Can you work these out from the model? Positions are in its coordinate system, mm. A direction names the side the tool comes from. Round coordinates to 2 decimals unless told otherwise and drop trailing zeros. Loops run counter-clockwise (first coordinate to the right, second up) from the corner with the lowest first, then second, coordinate; pieces in that order, holes last. Notation, with made-up numbers: (-13.5, 20.25) -> (-7.5, 20.25) arc R20 ccw to (-7.5, 57.25) -> close; hole circle Ø2 at (41, 10.5). An arc over 180 degrees is marked (long way). Use a Markdown table: item, result.
from build123d import *

# Parameters (mm, degrees)
SALIENTE_EXTRUIR1_DEPTH      = 6
SALIENTE_EXTRUIR1_DEPTH_BACK = 6
CROQUIS3_R                   = 2.5
SALIENTE_EXTRUIR2_DEPTH      = 4.5
CROQUIS4_R                   = 2.4
SALIENTE_EXTRUIR5_DEPTH      = 7.5
CORTAR_EXTRUIR1_DEPTH        = 3.5


with BuildPart() as part:
    # Croquis1 → Saliente-Extruir1 (new, two sides: drawn at the far end of the back side and taken through both)
    with BuildSketch(Plane.XY.offset(-SALIENTE_EXTRUIR1_DEPTH_BACK)):
        Polygon((-11.5, 7), (-16.5, 7), (-16.5, 4.5), (-11.5, 4.5), (-11.5, -11.5), (11.5, -11.5), (11.5, 4.5), (16.5, 4.5), (16.5, 7), (11.5, 7), (11.5, 11.5), (-11.5, 11.5), align=None)
    extrude(amount=SALIENTE_EXTRUIR1_DEPTH + SALIENTE_EXTRUIR1_DEPTH_BACK)

    # Croquis3 → Saliente-Extruir2 (add)
    with BuildSketch(Plane(origin=(0, 11.5, 0), x_dir=(1, 0, 0), z_dir=(0, 1, 0))):
        with BuildLine():
            Line((0.5, 2.5), (-0.045643943, 2.5))
            ThreePointArc((-0.045643943, 2.5), (-11.5, 0), (-0.045643943, -2.5))
            Line((-0.045643943, -2.5), (0.5, -2.5))
            ThreePointArc((0.5, -2.5), (3, 0), (0.5, 2.5))
        make_face()
        with Locations(Location((-5.5, 0, 0), (0, 0, 270))):
            Circle(CROQUIS3_R, mode=Mode.SUBTRACT)
    extrude(amount=SALIENTE_EXTRUIR2_DEPTH)

    # Croquis4 → Saliente-Extruir5 (add)
    with BuildSketch(Plane(origin=(0, 11.5, 0), x_dir=(1, 0, 0), z_dir=(0, 1, 0))):
        with Locations(Location((-5.5, 0, 0), (0, 0, 270))):
            Circle(CROQUIS4_R)
    extrude(amount=SALIENTE_EXTRUIR5_DEPTH)

    # Croquis6 → Cortar-Extruir1 (cut)
    with BuildSketch(Plane(origin=(0, 7, 0), x_dir=(1, 0, 0), z_dir=(0, 1, 0))):
        with BuildLine():
            Line((-16.5, 0.59249524), (-16.5, -0.535898385))
            Line((-16.5, -0.535898385), (-15.434038365, -0.250274826))
            ThreePointArc((-15.434038365, -0.250274826), (-13.489741501, 0.12166281), (-15.45994605, 0.313813624))
            Line((-15.45994605, 0.313813624), (-16.5, 0.59249524))
        make_face()
        with BuildLine():
            Line((15.465925826, 0.258819045), (16.5, 0.535898385))
            Line((16.5, 0.535898385), (16.5, -0.535898385))
            Line((16.5, -0.535898385), (15.465925826, -0.258819045))
            ThreePointArc((15.465925826, -0.258819045), (13.5, 0), (15.465925826, 0.258819045))
        make_face()
    extrude(amount=-CORTAR_EXTRUIR1_DEPTH, mode=Mode.SUBTRACT)


solid = part.part
1. Which directions (+Z, -Z, +X, -X, +Y, -Y) give clear straight access to the entire face, cutting with the end or side of a thin tool? Please do faces 5 (the flat face through (13, 4.5, 0)), 6 (the flat face through (-2.7, 16, -0.1)), 7 (the flat face through (16, 5.8, 0.4)).
Answer sheet:
| item | result |
|---|---|
| face 5 | +Z, -Z, +X, -Y |
| face 6 | +Y |
| face 7 | +X, +Y, -Y |
2. If we mould it in two halves opening along X, with no side actions, what happens to faces 1 (the cylindrical face through (3, 14, 0)), 2 (the cylindrical face through (-13.49, 5.77, -0.08)), 3 (the flat face through (-13, 7, 0)), 4 (the cylindrical face through (13.5, 5.8, 0))? For each: +X half, -X half, draft (parallel to the pull), parting line (faces both ways), or undercut.
Answer sheet:
| item | result |
|---|---|
| face 1 | +X half |
| face 2 | undercut |
| face 3 | draft |
| face 4 | undercut |
3. I want a section at D-D (x = -12). Please give me the cut outline in (y, z), plus the area to 3 significant figures.
Answer sheet:
| item | result |
|---|---|
| outline | (4.5, -6) -> (7, -6) -> (7, 6) -> (4.5, 6) -> close |
| area | 30.0 mm² |
4. I want a section at C-C (y = -7). Please give me the cut outline in (x, z).
Answer sheet:
| item | result |
|---|---|
| outline | (-11.5, -6) -> (11.5, -6) -> (11.5, 6) -> (-11.5, 6) -> close |
5. Will these pins go through, and if not, where does the flat tip stop? pin 1 Ø1 at (y, z) = (2.5, -3.5) entering from -X; pin 2 Ø2.5 at (x, z) = (-14, -2.5) entering from +Y; pin 3 Ø5.5 at (x, z) = (14, 1.5) entering from +Y.
Answer sheet:
| item | result |
|---|---|
| pin 1 | stops at x = -11.5 |
| pin 2 | stops at y = 7 |
| pin 3 | stops at y = 11.5 |
6. I want a section at A-A (x = 14.5). Please give me the cut outline in (y, z).
Answer sheet:
| item | result |
|---|---|
| outline | (4.5, -6) -> (7, -6) -> (7, -1) -> (4.5, -1) -> close; (4.5, 1) -> (7, 1) -> (7, 6) -> (4.5, 6) -> close |
7. I need wall thicknesses on line 1 (Z direction, x = 14.5, y = 6.05); line 2 (X direction, y = 5, z = 0.75); line 3 (X direction, y = -10, z = 4.5). Which ranges of each line are inside material? Lowest first, please.
Answer sheet:
| item | result |
|---|---|
| line 1 | z = -6 to -1, 1 to 6 |
| line 2 | x = -16.5 to -15.05, -13.92 to 13.84, 15.16 to 16.5 |
| line 3 | x = -11.5 to 11.5 |
8. I want a section at B-B (z = -1.5). Please give me the cut outline in (x, y).
Answer sheet:
| item | result |
|---|---|
| outline | (-16.5, 4.5) -> (-11.5, 4.5) -> (-11.5, -11.5) -> (11.5, -11.5) -> (11.5, 4.5) -> (16.5, 4.5) -> (16.5, 7) -> (11.5, 7) -> (11.5, 11.5) -> (2.5, 11.5) -> (2.5, 16) -> (-3.5, 16) -> (-3.5, 11.5) -> (-3.63, 11.5) -> (-3.63, 19) -> (-7.37, 19) -> (-7.37, 11.5) -> (-7.5, 11.5) -> (-7.5, 16) -> (-11.31, 16) -> (-11.31, 11.5) -> (-11.5, 11.5) -> (-11.5, 7) -> (-16.5, 7) -> close |
